```python
from build123d import *

# Parameters (mm, degrees)
SKETCH1_W           = 66.5
SKETCH1_H           = 46.5
BOSS_EXTRUDE1_DEPTH = 3
SKETCH2_W           = 60.5
SKETCH2_H           = 42.5
BOSS_EXTRUDE2_DEPTH = 4
SKETCH3_R           = 13.2
CUT_EXTRUDE1_DEPTH  = 4
SKETCH4_R           = 2.25
CUT_EXTRUDE2_DEPTH  = 4
SKETCH5_R           = 4.5
CUT_EXTRUDE3_DEPTH  = 1
SKETCH6_R           = 17.2
SKETCH6_R_2         = 13.2
BOSS_EXTRUDE3_DEPTH = 6
FILLET1_R           = 1
CHAMFER1_SIZE       = 2
SKETCH7_W           = 3
SKETCH7_H           = 16.5
BOSS_EXTRUDE4_DEPTH = 21.5
SKETCH8_W           = 16.5
SKETCH8_H           = 3
BOSS_EXTRUDE5_DEPTH = 1.5
SKETCH9_W           = 16.5
SKETCH9_H           = 3
BOSS_EXTRUDE6_DEPTH = 1.5
CHAMFER2_SIZE       = 2
CHAMFER3_SIZE       = 2
CHAMFER4_SIZE       = 2
CHAMFER5_SIZE       = 5
CHAMFER6_SIZE       = 5
BOSS_EXTRUDE7_START = -2
SKETCH10_R          = 13.2
SKETCH10_R_2        = 9
BOSS_EXTRUDE7_DEPTH = 2


with BuildPart() as part:
    # Sketch1 → Boss-Extrude1 (new body)
    with BuildSketch(Plane(origin=(0, 0, 0), x_dir=(1, 0, 0), z_dir=(0, 1, 0))):
        with Locations((0.065324165, -4.697937132)):
            Rectangle(SKETCH1_W, SKETCH1_H)
    extrude(amount=BOSS_EXTRUDE1_DEPTH)

    # Sketch2 → Boss-Extrude2 (add)
    with BuildSketch(Plane(origin=(0, 3, 0), x_dir=(1, 0, 0), z_dir=(0, 1, 0))):
        Polygon((-30.184675835, 18.552062868), (-33.184675835, 18.552062868), (-33.184675835, 16.552062868), (-33.184675835, -25.947937132), (-33.184675835, -27.947937132), (-30.184675835, -27.947937132), (30.315324165, -27.947937132), (33.315324165, -27.947937132), (33.315324165, -25.947937132), (33.315324165, 16.552062868), (33.315324165, 18.552062868), (30.315324165, 18.552062868), align=None)
        with Locations((0.065324165, -4.697937132)):
            Rectangle(SKETCH2_W, SKETCH2_H, mode=Mode.SUBTRACT)
    extrude(amount=BOSS_EXTRUDE2_DEPTH)

    # Sketch3 → Cut-Extrude1 (cut)
    with BuildSketch(Plane(origin=(0, 3, 0), x_dir=(1, 0, 0), z_dir=(0, 1, 0))):
        with Locations(Location((12.915324165, -4.697937132, 0), (0, 0, 270))):
            Circle(SKETCH3_R)
    extrude(amount=-CUT_EXTRUDE1_DEPTH, mode=Mode.SUBTRACT)

    # Sketch4 → Cut-Extrude2 (cut)
    with BuildSketch(Plane(origin=(0, 3, 0), x_dir=(1, 0, 0), z_dir=(0, 1, 0))):
        with Locations(Location((-15.184675835, -4.697937132, 0), (0, 0, 270))):
            Circle(SKETCH4_R)
    extrude(amount=-CUT_EXTRUDE2_DEPTH, mode=Mode.SUBTRACT)

    # Sketch5 → Cut-Extrude3 (cut)
    with BuildSketch(Plane(origin=(0, 3, 0), x_dir=(1, 0, 0), z_dir=(0, 1, 0))):
        with Locations(Location((-15.184675835, -4.697937132, 0), (0, 0, 270))):
            Circle(SKETCH5_R)
    extrude(amount=-CUT_EXTRUDE3_DEPTH, mode=Mode.SUBTRACT)

    # Sketch6 → Boss-Extrude3 (add)
    with BuildSketch(Plane.XZ):
        with Locations(Location((12.915324165, 4.697937132, 0), (0, 0, 90))):
            Circle(SKETCH6_R)
        with Locations(Location((12.915324165, 4.697937132, 0), (0, 0, 90))):
            Circle(SKETCH6_R_2, mode=Mode.SUBTRACT)
    extrude(amount=BOSS_EXTRUDE3_DEPTH)

    # Fillet1
    fillet1_edges = [part.edges().sort_by_distance(p)[0] for p in [
        (-30.184675835, 5, -16.552062868),
        (30.315324165, 5, -16.552062868),
        (30.315324165, 5, 25.947937132),
        (-30.184675835, 5, 25.947937132),
    ]]
    fillet(fillet1_edges, radius=FILLET1_R)

    # Chamfer1
    chamfer1_edges = [part.edges().sort_by_distance(p)[0] for p in [
        (-33.184675835, 3.5, -18.552062868),
        (33.315324165, 3.5, -18.552062868),
        (33.315324165, 3.5, 27.947937132),
        (-33.184675835, 3.5, 27.947937132),
    ]]
    chamfer(chamfer1_edges, length=CHAMFER1_SIZE)

    # Sketch7 → Boss-Extrude4 (add)
    with BuildSketch(Plane(origin=(0, 7, 0), x_dir=(1, 0, 0), z_dir=(0, 1, 0))):
        with Locations((31.815324165, -4.697937132)):
            Rectangle(SKETCH7_W, SKETCH7_H)
        with Locations((-31.684675835, -4.697937132)):
            Rectangle(SKETCH7_W, SKETCH7_H)
    extrude(amount=BOSS_EXTRUDE4_DEPTH)

    # Sketch8 → Boss-Extrude5 (add)
    with BuildSketch(Plane.ZY.offset(-30.315324165)):
        with Locations((4.697937132, 27)):
            Rectangle(SKETCH8_W, SKETCH8_H)
    extrude(amount=BOSS_EXTRUDE5_DEPTH)

    # Sketch9 → Boss-Extrude6 (add)
    with BuildSketch(Plane(origin=(-30.184675835, 0, 0), x_dir=(0, 0, -1), z_dir=(1, 0, 0))):
        with Locations((-4.697937132, 27)):
            Rectangle(SKETCH9_W, SKETCH9_H)
    extrude(amount=BOSS_EXTRUDE6_DEPTH)

    # Chamfer2
    chamfer2_edges = [part.edges().sort_by_distance(p)[0] for p in [
        (28.815324165, 28.5, 4.697937132),
        (-28.684675835, 28.5, 4.697937132),
    ]]
    chamfer(chamfer2_edges, length=CHAMFER2_SIZE)

    # Chamfer3
    chamfer3_edges = [part.edges().sort_by_distance(p)[0] for p in [
        (12.915324165, 3, -8.502062868),
    ]]
    chamfer(chamfer3_edges, length=CHAMFER3_SIZE)

    # Chamfer4
    chamfer4_edges = [part.edges().sort_by_distance(p)[0] for p in [
        (12.915324165, 0, -12.502062868),
    ]]
    chamfer(chamfer4_edges, length=CHAMFER4_SIZE)

    # Chamfer5
    chamfer5_edges = [part.edges().sort_by_distance(p)[0] for p in [
        (31.815324165, 7, -3.552062868),
        (31.815324165, 7, 12.947937132),
    ]]
    chamfer(chamfer5_edges, length=CHAMFER5_SIZE)

    # Chamfer6
    chamfer6_edges = [part.edges().sort_by_distance(p)[0] for p in [
        (-31.684675835, 7, -3.552062868),
        (-31.684675835, 7, 12.947937132),
    ]]
    chamfer(chamfer6_edges, length=CHAMFER6_SIZE)

    # Sketch10 → Boss-Extrude7 (add)
    with BuildSketch(Plane.XZ.offset(6).offset(BOSS_EXTRUDE7_START)):
        with Locations(Location((12.915324165, 4.697937132, 0), (0, 0, 90))):
            Circle(SKETCH10_R)
        with Locations(Location((12.915324165, 4.697937132, 0), (0, 0, 270))):
            Circle(SKETCH10_R_2, mode=Mode.SUBTRACT)
    extrude(amount=BOSS_EXTRUDE7_DEPTH)


solid = part.part
```
Check sheet for the modelled part. Datum: model origin and axes. Units: mm. A direction names the side the tool comes from. Coordinates: 2 decimals unless noted, no trailing zeros. Write each loop counter-clockwise with the first axis right and the second up, starting at its lowest first coordinate (ties: lowest second). Pieces come first, ordered by that corner, then holes. Notation, with made-up numbers: M 34.25,49 L 68.25,49 A22 ccw 68.25,65 Z; hole C -14.75,-35.5 d1. An arc over 180 degrees is marked long. Use one line per item in the form item = value.
Item 1: Release check for a two-part mould opening along X. For faces 1 (the face through (-32.17, 3.45, 26.96)), 2 (the face through (-13, 2, 6)), 3 (the face through (-31.71, 9.54, 15.41)) record: pulls with the +X half, pulls with the -X half, needs draft (parallel to the pull), parting line crosses it, or undercut.
Answer below:
face_1 = pulls with the -X half
face_2 = undercut
face_3 = needs draft
Item 2: Sectioned sample at A-A, the plane y = 21.5. Record the cut outline in (x, z).
Answer below:
outline = M -33.18,-3.55 L -30.18,-3.55 L -30.18,12.95 L -33.18,12.95 Z; M 30.32,-3.55 L 33.32,-3.55 L 33.32,12.95 L 30.32,12.95 Z
Item 3: Sectioned sample at C-C, the plane x = -11.5. Record the cut outline in (y, z).
Answer below:
outline = M 0,-18.55 L 7,-18.55 L 7,-16.55 L 3,-16.55 L 3,2.11 L 2,2.11 L 2,7.28 L 3,7.28 L 3,25.95 L 7,25.95 L 7,27.95 L 0,27.95 Z
Item 4: Gauge pin test, flat ends, axial feed: pin 1 Ø10 at (x, z) = (-15, 3) entering from +Y; pin 2 Ø1.6 at (x, z) = (-29.5, 3.5) entering from -Y. Record the tip position at first contact, or that the pin passes through.
Answer below:
pin_1 = 3
pin_2 = 0
Item 5: Set-up check for faces 4 (the face through (0, 7, -17)), 5 (the face through (-29.671, 27.486, 4.813)), 6 (the face through (-30.185, 12, 5)), 7 (the face through (0, 5, 25.948)): record each of +Z, -Z, +X, -X, +Y, -Y from which the full face is reachable in a straight line by a thin tool's end or side.
Answer below:
face_4 = -Z, +X, -X, +Y
face_5 = +Z, -Z, +Y
face_6 = none
face_7 = +Y
Item 6: Sectioned sample at B-B, the plane x = -21. Record the cut outline in (y, z), and give its area (4 significant figures).
Answer below:
outline = M 0,-18.55 L 7,-18.55 L 7,-16.55 L 3,-16.55 L 3,25.95 L 7,25.95 L 7,27.95 L 0,27.95 Z
area = 155.5 mm^2
Item 7: Material ranges on L1, parallel to Z at x = 20.5, y = 5; L2, parallel to X at y = 20.5, z = 11.5; L3, parallel to Y at x = -19, z = 22.5, recorded low to high. Write a range as from..to.
Answer below:
L1 = -18.55..-16.55, 25.95..27.95
L2 = -33.18..-30.18, 30.32..33.32
L3 = 0..3
